Input: dimensioned drawing with shaded views. Units: mm. Origin: part minimum x, y, z. A direction names the side the tool comes from. Coordinates: 2 decimals unless noted, no trailing zeros. Order: outer loops, then holes, each group sorted by start corner. A loop starts at its lowest first (then second) coordinate and runs counter-clockwise, first axis right, second up.
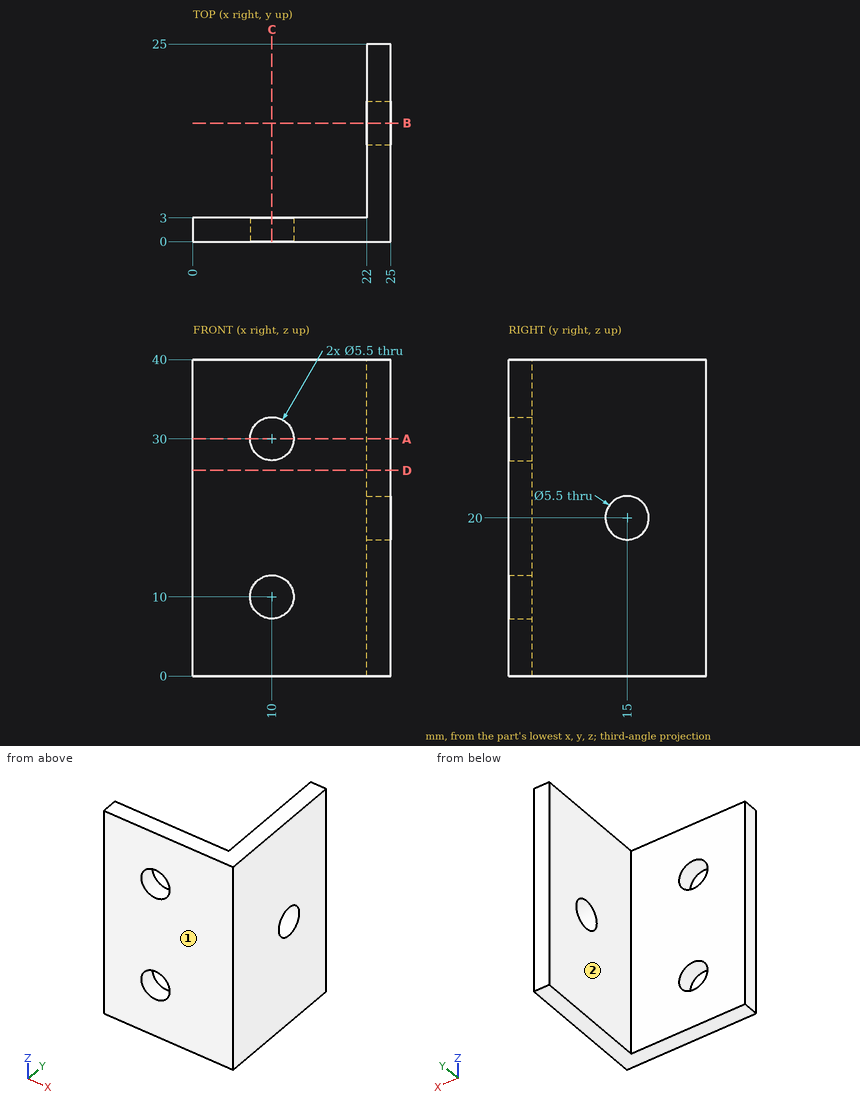
1. Access query for the marked faces 1 and 2. Directions: +Z, -Z, +X, -X, +Y, -Y. A direction counts if a zero-diameter tool reaches every point of the face in a straight line with its end or side. Return the directions, or none.
2. Section query B-B, the plane y = 15. Output: boundary loops of the cut face in (x, z).
3. Contact query for flat-ended pins moving along their axis: P1, Ø12, axis at y = 11, z = 6, coming from the -X side; P2, Ø1, axis at x = 9.5, z = 34, coming from the +Y side; P3, Ø3.5, axis at y = 15, z = 20, coming from the +X side. Output: stop coordinate, or through.
4. Section query A-A, the plane z = 30. Output: boundary loops of the cut face in (x, y).
5. Material intervals for line 1 along Z through (x, y) = (10, 1.05); line 2 along Y through (x, z) = (12.5, 12); line 3 along Y through (x, z) = (24, 20), sorted ascending.
6. Section query D-D, the plane z = 26. Output: boundary loops of the cut face in (x, y), plus the area to 3 significant figures.
7. Section query C-C, the plane x = 10. Output: boundary loops of the cut face in (y, z), plus the area to 3 significant figures.
Answer key:
1. face 1: +Z, -Z, +X, -X, -Y
1. face 2: +Z, -Z, -X, +Y
2. outline: (22, 0) - (25, 0) - (25, 17.25) - (22, 17.25) - close; (22, 22.75) - (25, 22.75) - (25, 40) - (22, 40) - close
3. P1: stops at x = 22
3. P2: stops at y = 3
3. P3: passes through
4. outline: (0, 0) - (7.25, 0) - (7.25, 3) - (0, 3) - close; (12.75, 0) - (25, 0) - (25, 25) - (22, 25) - (22, 3) - (12.75, 3) - close
5. line 1: z = 0 to 7.25, 12.75 to 27.25, 32.75 to 40
5. line 2: y = 0 to 3
5. line 3: y = 0 to 12.25, 17.75 to 25
6. outline: (0, 0) - (25, 0) - (25, 25) - (22, 25) - (22, 3) - (0, 3) - close
6. area: 141 mm2
7. outline: (0, 0) - (3, 0) - (3, 7.25) - (0, 7.25) - close; (0, 12.75) - (3, 12.75) - (3, 27.25) - (0, 27.25) - close; (0, 32.75) - (3, 32.75) - (3, 40) - (0, 40) - close
7. area: 87.0 mm2
